Part model, mm, in its own coordinate system. Face numbers are marked on the shaded views. A direction names the side the tool comes from. Give positions to 0.01 mm unless a question says otherwise; leave off trailing zeros. Order: outer loops, then holes, each group sorted by start corner. A loop starts at its lowest first (then second) coordinate and runs counter-clockwise, first axis right, second up. Notation, with made-up numbers: (78.5, -15) - (111.5, -15) arc R20 cw to (111.5, 4) - close; hole circle Ø5 at (-23.5, 54.25). An arc over 180 degrees is marked (long way). Use a Markdown table: item, result. Add a question column.
from build123d import *

# Parameters (mm, degrees)
BASE_FLANGE1_DEPTH = 490.75


# Sheet-metal steps are written as plain solids
with BuildPart() as part:
    # Sketch1 → Base-Flange1 (new, symmetric)
    with BuildSketch(Plane(origin=(0, 0, 0), x_dir=(1, 0, 0), z_dir=(0, 1, 0))):
        with BuildLine():
            Line((9.5, 55.75), (9.5, 67.7634))
            ThreePointArc((9.5, 67.7634), (10.081861668, 69.168138332), (11.4866, 69.75))
            Line((11.4866, 69.75), (37.5134, 69.75))
            ThreePointArc((37.5134, 69.75), (38.918138332, 69.168138332), (39.5, 67.7634))
            Line((39.5, 67.7634), (39.5, 18.25))
            Line((39.5, 18.25), (39.5, 8.562771629))
            ThreePointArc((39.5, 8.562771629), (39.724914644, 8.032905932), (40.262306969, 7.826620346))
            Line((40.262306969, 7.826620346), (42.153527557, 7.892663224))
            ThreePointArc((42.153527557, 7.892663224), (42.675221066, 8.135932903), (42.862626267, 8.680197126))
            Line((42.862626267, 8.680197126), (42.359529101, 15.874821789))
            ThreePointArc((42.359529101, 15.874821789), (42.88838258, 17.368257942), (44.341289843, 18))
            Line((44.341289843, 18), (53.5134, 18))
            ThreePointArc((53.5134, 18), (54.918138332, 17.418138332), (55.5, 16.0134))
            Line((55.5, 16.0134), (55.5, -20.75))
            Line((55.5, -20.75), (55.5, -65.7634))
            ThreePointArc((55.5, -65.7634), (54.918138332, -67.168138332), (53.5134, -67.75))
            Line((53.5134, -67.75), (39.5, -67.75))
            Line((39.5, -67.75), (11.4866, -67.75))
            ThreePointArc((11.4866, -67.75), (10.081861668, -67.168138332), (9.5, -65.7634))
            Line((9.5, -65.7634), (9.5, -53.75))
            Line((9.5, -53.75), (10.75, -53.75))
            Line((10.75, -53.75), (10.75, -65.7634))
            ThreePointArc((10.75, -65.7634), (10.965745145, -66.284254855), (11.4866, -66.5))
            Line((11.4866, -66.5), (39.5, -66.5))
            Line((39.5, -66.5), (53.5134, -66.5))
            ThreePointArc((53.5134, -66.5), (54.034254855, -66.284254855), (54.25, -65.7634))
            Line((54.25, -65.7634), (54.25, -20.75))
            Line((54.25, -20.75), (54.25, 16.0134))
            ThreePointArc((54.25, 16.0134), (54.034254855, 16.534254855), (53.5134, 16.75))
            Line((53.5134, 16.75), (44.341289843, 16.75))
            ThreePointArc((44.341289843, 16.75), (43.802574707, 16.515759992), (43.606484164, 15.962017381))
            Line((43.606484164, 15.962017381), (44.10958133, 8.767392718))
            ThreePointArc((44.10958133, 8.767392718), (43.604152098, 7.299519645), (42.197151928, 6.64342469))
            Line((42.197151928, 6.64342469), (40.30593134, 6.577381812))
            ThreePointArc((40.30593134, 6.577381812), (38.856591681, 7.133731182), (38.25, 8.562771629))
            Line((38.25, 8.562771629), (38.25, 18.25))
            Line((38.25, 18.25), (38.25, 67.7634))
            ThreePointArc((38.25, 67.7634), (38.034254855, 68.284254855), (37.5134, 68.5))
            Line((37.5134, 68.5), (11.4866, 68.5))
            ThreePointArc((11.4866, 68.5), (10.965745145, 68.284254855), (10.75, 67.7634))
            Line((10.75, 67.7634), (10.75, 55.75))
            Line((10.75, 55.75), (9.5, 55.75))
        make_face()
    extrude(amount=BASE_FLANGE1_DEPTH, both=True)


solid = part.part
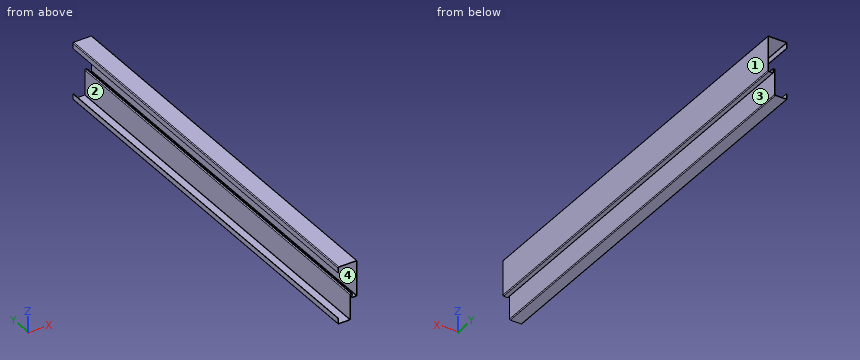
1. Mould opens along Z. For the marked faces 3 and 4 say: released by +Z, released by -Z, zero draft, split by the parting line, or undercut.
2. Cut at A-A (x = 23.5). Write the cut outline in (y, z), plus the area to 3 significant figures.
3. Cut at B-B (z = 10). Write the cut outline in (x, y).
4. Drill centre lines: probe 1 along Z at (x, y) = (14, 397); probe 2 along Z at (x, y) = (41.5, 161.5); probe 3 along X at (y, z) = (157, 32.5). Where is each one in solid material? Low to high. Write a range as [from, to].
5. Pin check, flat tips, straight feed: P1, Ø1, axis at x = 10, y = -244, coming from the -Z side; P2, Ø9.5, axis at y = 221, z = -60.5, coming from the +X side; P3, Ø6, axis at y = -136.5, z = -21, coming from the -X side. Stop position of each tip, or through.
6. Tool access for the marked faces 1 and 2: list every direction of +Z, -Z, +X, -X, +Y, -Y with a clear straight run to the whole face (end or side of a thin tool).
Responses:
| question | item | result |
|---|---|---|
| 1 | face 3 | zero draft |
| 1 | face 4 | undercut |
| 2 | outline | (-490.75, -69.75) - (490.75, -69.75) - (490.75, -68.5) - (-490.75, -68.5) - close; (-490.75, 66.5) - (490.75, 66.5) - (490.75, 67.75) - (-490.75, 67.75) - close |
| 2 | area | 2,450 mm² |
| 3 | outline | (54.25, -490.75) - (55.5, -490.75) - (55.5, 490.75) - (54.25, 490.75) - close |
| 4 | probe 1 | z = [-69.75, -68.5], [66.5, 67.75] |
| 4 | probe 2 | z = [-7.87, -6.62], [66.5, 67.75] |
| 4 | probe 3 | x = [54.25, 55.5] |
| 5 | P1 | stops at z = -69.49 |
| 5 | P2 | stops at x = 39.5 |
| 5 | P3 | stops at x = 38.25 |
| 6 | face 1 | +Z, -Z, +X, +Y, -Y |
| 6 | face 2 | +Y, -Y |
